from build123d import *

# Parameters (mm, degrees)
ESBO_O1_W                = 31
ESBO_O1_H                = 40
RESSALTO_EXTRUS_O1_DEPTH = 6
ESBO_O2_R                = 2
ESBO_O2_W                = 5
ESBO_O2_H                = 25
CORTE_EXTRUS_O1_DEPTH    = 6
ESBO_O4_R                = 1.5
CORTE_EXTRUS_O2_DEPTH    = 6
ESBO_O5_R                = 2.5
CORTE_EXTRUS_O3_DEPTH    = 2.4
FILETE1_R                = 5


with BuildPart() as part:
    # Esboço1 → Ressalto-extrusão1 (new body)
    with BuildSketch(Plane.XY):
        Rectangle(ESBO_O1_W, ESBO_O1_H)
    extrude(amount=RESSALTO_EXTRUS_O1_DEPTH)

    # Esboço2 → Corte-extrusão1 (cut)
    with BuildSketch(Plane.XY.offset(6)):
        with Locations((-5.5, -12)):
            Circle(ESBO_O2_R)
        with Locations((-5.5, 0)):
            Circle(ESBO_O2_R)
        with Locations((13, -7.5)):
            Rectangle(ESBO_O2_W, ESBO_O2_H)
    extrude(amount=-CORTE_EXTRUS_O1_DEPTH, mode=Mode.SUBTRACT)

    # Esboço4 → Corte-extrusão2 (cut)
    with BuildSketch(Plane.XY.offset(6)):
        with Locations((0.8125, 13.4375)):
            Circle(ESBO_O4_R)
        with Locations((10.3375, 13.4375)):
            Circle(ESBO_O4_R)
    extrude(amount=-CORTE_EXTRUS_O2_DEPTH, mode=Mode.SUBTRACT)

    # Esboço5 → Corte-extrusão3 (cut)
    with BuildSketch(Plane(origin=(0, 0, 0), x_dir=(-1, 0, 0), z_dir=(0, 0, -1))):
        with Locations((-0.8125, 13.4375)):
            Circle(ESBO_O5_R)
        with Locations((-10.3375, 13.4375)):
            Circle(ESBO_O5_R)
    extrude(amount=-CORTE_EXTRUS_O3_DEPTH, mode=Mode.SUBTRACT)

    # Filete1
    filete1_edges = [part.edges().sort_by_distance(p)[0] for p in [
        (10.5, 5, 3),
    ]]
    fillet(filete1_edges, radius=FILETE1_R - 0.0001)  # a hair under: the kernel refuses the full size


solid = part.part
For this review, take the finished solid that the model builds, in its own axes (mm). A direction names the side the tool comes from. Coordinates: 2 decimals unless noted, no trailing zeros. Order: outer loops, then holes, each group sorted by start corner. A loop starts at its lowest first (then second) coordinate and runs counter-clockwise, first axis right, second up. Notation, with made-up numbers: (17.25, 14) - (21.25, 14) arc R13 ccw to (21.25, 33) - close; hole circle Ø9 at (48.25, -21). An arc over 180 degrees is marked (long way). Answer as CSV lines item,"result". Start each with the question number.
1) Draft analysis for pull direction X (two halves, no side actions). For faces 1 (the cylindrical face through (1.354, 10.997, 1.183)), 2 (the flat face through (0, 20, 3)), 3 (the flat face through (-15.5, 0, 3)), state which applies: +X half, -X half, draft (parallel to the pull), parting line (faces both ways), or undercut.
2) Add section B-B (z = 1.25). Count the separate pieces of the cut face and the enclosed holes in it, then the cut area to 3 significant figures.
3) Insertion check: P1, Ø2.5, axis at x = 0.81, y = 13.44, coming from the +Z side; P2, Ø2, axis at y = -3.5, z = 2.5, coming from the +X side. Each pin has a flat end and moves straight along its axis. Give the tip position at first contact, or say it passes through.
4) Add section C-C (x = 11). State the section outline as (y, z) points, then the cut area to 3 significant figures.
5) To check wall thickness, follow line 1 along Y through (x, z) = (-5.5, 3.45); line 2 along X through (y, z) = (13.5, 1.45); line 3 along Y through (x, z) = (-4, 2.1). State the ranges of each line that lie inside material, in increasing order. Write a range as [from, to].
6) Add section D-D (x = -7). State the section outline as (y, z) points, then the cut area to 3 significant figures.
7) Add section A-A (y = -12). State the section outline as (x, z) points, then the cut area to 3 significant figures.
8) Machinability: for faces 4 (the flat face through (10.5, -10, 3)), 5 (the flat face through (0, 0, 6)), 6 (the cylindrical face through (10.9, 11, 1.2)), which of the approach directions +Z, -Z, +X, -X, +Y, -Y give a long, thin tool a straight path to every point of the face, cutting with its end or side? Answer none if there is none.
Result:
1,face 1,"undercut"
1,face 2,"draft"
1,face 3,"-X half"
2,separate pieces,"1"
2,enclosed holes,"4"
2,area,"1,060 mm^2"
3,P1,"through"
3,P2,"x = 10.5"
4,outline,"(2.18, 0) - (11.03, 0) - (11.03, 2.4) - (12.09, 2.4) - (12.09, 6) - (2.18, 6) - close; (14.78, 2.4) - (15.85, 2.4) - (15.85, 0) - (20, 0) - (20, 6) - (14.78, 6) - close"
4,area,"85.7 mm^2"
5,line 1,"[-20, -14], [-10, -2], [2, 20]"
5,line 2,"[-15.5, -1.69], [3.31, 7.84], [12.84, 15.5]"
5,line 3,"[-20, -13.32], [-10.68, -1.32], [1.32, 20]"
6,outline,"(-20, 0) - (-13.32, 0) - (-13.32, 6) - (-20, 6) - close; (-10.68, 0) - (-1.32, 0) - (-1.32, 6) - (-10.68, 6) - close; (1.32, 0) - (20, 0) - (20, 6) - (1.32, 6) - close"
6,area,"208 mm^2"
7,outline,"(-15.5, 0) - (-7.5, 0) - (-7.5, 6) - (-15.5, 6) - close; (-3.5, 0) - (10.5, 0) - (10.5, 6) - (-3.5, 6) - close"
7,area,"132 mm^2"
8,face 4,"+Z, -Z, +X, -Y"
8,face 5,"+Z, +X, -X, +Y, -Y"
8,face 6,"-Z"
